Check sheet for the modelled part. Datum: model origin and axes. Units: mm. Give positions to 0.01 mm unless a question says otherwise; leave off trailing zeros. Write each loop counter-clockwise with the first axis right and the second up, starting at its lowest first coordinate (ties: lowest second). Pieces come first, ordered by that corner, then holes. Notation, with made-up numbers: (54, 56.25) -> (61, 56.25) arc R28 cw to (61, 80.25) -> close; hole circle Ø1 at (74, 40). An arc over 180 degrees is marked (long way). Return JSON: item names as keys, results as strings.
from build123d import *

# Parameters (mm, degrees)
BOSS_EXTRUDE1_DEPTH = 5
SKETCH3_R           = 0.75
CUT_EXTRUDE1_DEPTH  = 3
SKETCH4_R           = 0.75
CUT_EXTRUDE2_DEPTH  = 3


with BuildPart() as part:
    # Sketch2 → Boss-Extrude1 (new body)
    with BuildSketch(Plane(origin=(0, 0, 0), x_dir=(1, 0, 0), z_dir=(0, 1, 0))):
        with BuildLine():
            Line((-27.42, 36), (-27.42, 8.582019714))
            Line((-27.42, 8.582019714), (-27.42, -8.582019714))
            Line((-27.42, -8.582019714), (-27.42, -36))
            ThreePointArc((-27.42, -36), (-36, -44.58), (-44.58, -36))
            Line((-44.58, -36), (-44.58, -8.582019714))
            Line((-44.58, -8.582019714), (-44.58, 8.582019714))
            Line((-44.58, 8.582019714), (-44.58, 36))
            ThreePointArc((-44.58, 36), (-36, 44.58), (-27.42, 36))
        make_face()
    extrude(amount=BOSS_EXTRUDE1_DEPTH)

    # Sketch3 → Cut-Extrude1 (cut)
    with BuildSketch(Plane.XZ):
        with Locations((-36, 0)):
            Circle(SKETCH3_R)
    extrude(amount=-CUT_EXTRUDE1_DEPTH, mode=Mode.SUBTRACT)

    # Sketch4 → Cut-Extrude2 (cut)
    with BuildSketch(Plane(origin=(0, 5, 0), x_dir=(1, 0, 0), z_dir=(0, 1, 0))):
        with Locations((-36, 36)):
            Circle(SKETCH4_R)
        with Locations((-36, -36)):
            Circle(SKETCH4_R)
    extrude(amount=-CUT_EXTRUDE2_DEPTH, mode=Mode.SUBTRACT)


solid = part.part
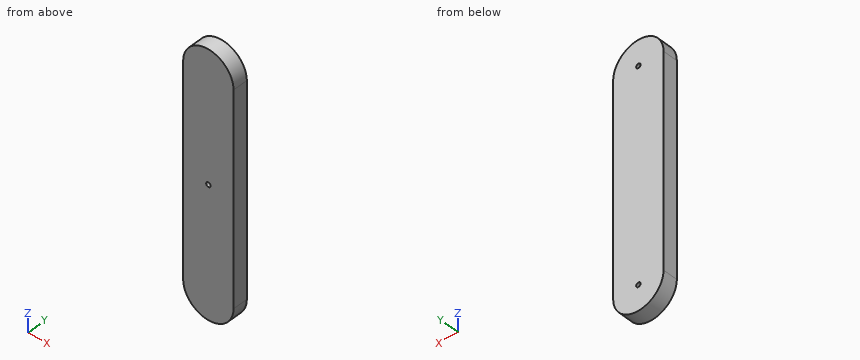
(1) Depth check by flat-ended pin: pin 1 Ø0.8 at (x, z) = (-36, 0) entering from -Y; pin 2 Ø2 at (x, z) = (-32, -27.5) entering from -Y. Enter the tip coordinate at first touch or a pass-through.
Reply:
{"pin 1": "y = 3", "pin 2": "y = 0"}
(2) Thickness scan on L1, parallel to Z at x = -36, y = 3.75; L2, parallel to X at y = 3.1, z = 36; L3, parallel to Z at x = -33.5, y = 2.8. Record the ranges inside material, lowest first.
Reply:
{"L1": "-44.58 to -36.75, -35.25 to 35.25, 36.75 to 44.58", "L2": "-44.58 to -36.75, -35.25 to -27.42", "L3": "-44.21 to 44.21"}
(3) Cross-section at B-B on x = -36. Enter the section's corners in (y, z), then the cut area to 3 significant figures.
Reply:
{"outline": "(0, -44.58) -> (5, -44.58) -> (5, -36.75) -> (2, -36.75) -> (2, -35.25) -> (5, -35.25) -> (5, 35.25) -> (2, 35.25) -> (2, 36.75) -> (5, 36.75) -> (5, 44.58) -> (0, 44.58) -> (0, 0.75) -> (3, 0.75) -> (3, -0.75) -> (0, -0.75) -> close", "area": "432 mm^2"}
(4) Cross-section at C-C on x = -40.25. Enter the section's corners in (y, z).
Reply:
{"outline": "(0, -43.45) -> (5, -43.45) -> (5, 43.45) -> (0, 43.45) -> close"}
(5) Cross-section at A-A on y = 4. Enter the section's corners in (x, z), then the cut area to 3 significant figures.
Reply:
{"outline": "(-44.58, -36) arc R8.58 ccw to (-27.42, -36) -> (-27.42, 36) arc R8.58 ccw to (-44.58, 36) -> close; hole circle Ø1.5 at (-36, -36); hole circle Ø1.5 at (-36, 36)", "area": "1,460 mm^2"}
(6) Cross-section at D-D on x = -29.5. Enter the section's corners in (y, z), then the cut area to 3 significant figures.
Reply:
{"outline": "(0, -41.6) -> (5, -41.6) -> (5, 41.6) -> (0, 41.6) -> close", "area": "416 mm^2"}
